from build123d import *

# Parameters (mm, degrees)
SKETCH1_W                               = 200
SKETCH1_H                               = 200
BOSS_EXTRUDE1_DEPTH                     = 8
CBORE_FOR_M2_PAN_HEAD_SCREW1_AT_2_COUNT = 2
CBORE_FOR_M2_PAN_HEAD_SCREW1_AT_2_PITCH = 89.990465529
CBORE_FOR_M2_PAN_HEAD_SCREW1_AT_3_COUNT = 2
CBORE_FOR_M2_PAN_HEAD_SCREW1_AT_3_PITCH = 89.990465529
CBORE_FOR_M2_PAN_HEAD_SCREW1_AT_4_COUNT = 2
CBORE_FOR_M2_PAN_HEAD_SCREW1_AT_4_PITCH = 66.987356945
CBORE_FOR_M2_PAN_HEAD_SCREW1_AT_5_COUNT = 2
CBORE_FOR_M2_PAN_HEAD_SCREW1_AT_5_PITCH = 23.002979742
SKETCH7_R                               = 2.5
CUT_EXTRUDE1_DEPTH                      = 4
SKETCH9_R                               = 1.5
CUT_EXTRUDE2_DEPTH                      = 10
LPATTERN1_COUNT                         = 2
LPATTERN1_PITCH                         = 100.5


with BuildPart() as part:
    # Sketch1 → Boss-Extrude1 (new body)
    with BuildSketch(Plane.XY):
        with Locations((100, 100)):
            Rectangle(SKETCH1_W, SKETCH1_H)
    extrude(amount=BOSS_EXTRUDE1_DEPTH)

    # Sketch6 → CBORE for M2 Pan Head Screw1 (revolve, cut)
    with BuildSketch(Plane(origin=(49.75, 55.009534471, 0), x_dir=(0, 1, 0), z_dir=(1, 0, 0))):
        Polygon((0, 0), (0, 8.901290929), (1.5, 8), (1.5, 4), (2.5, 4), (2.5, 0), align=None)
    cbore_for_m2_pan_head_screw1 = revolve(axis=Axis((49.75, 55.009534471, -6.35), (0, 0, 1)), mode=Mode.SUBTRACT)

    # CBORE for M2 Pan Head Screw1 at 2: CBORE for M2 Pan Head Screw1 ×2
    with Locations(*[(0, i * CBORE_FOR_M2_PAN_HEAD_SCREW1_AT_2_PITCH, 0) for i in range(1, CBORE_FOR_M2_PAN_HEAD_SCREW1_AT_2_COUNT)]):
        add(cbore_for_m2_pan_head_screw1, mode=Mode.SUBTRACT)

    # CBORE for M2 Pan Head Screw1 at 3: CBORE for M2 Pan Head Screw1 ×2
    with Locations(*[(0, i * CBORE_FOR_M2_PAN_HEAD_SCREW1_AT_3_PITCH, 0) for i in range(1, CBORE_FOR_M2_PAN_HEAD_SCREW1_AT_3_COUNT)]):
        add(cbore_for_m2_pan_head_screw1, mode=Mode.SUBTRACT)

    # CBORE for M2 Pan Head Screw1 at 4: CBORE for M2 Pan Head Screw1 ×2
    with Locations(*[(0, i * CBORE_FOR_M2_PAN_HEAD_SCREW1_AT_4_PITCH, 0) for i in range(1, CBORE_FOR_M2_PAN_HEAD_SCREW1_AT_4_COUNT)]):
        add(cbore_for_m2_pan_head_screw1, mode=Mode.SUBTRACT)

    # CBORE for M2 Pan Head Screw1 at 5: CBORE for M2 Pan Head Screw1 ×2
    with Locations(*[(0, i * CBORE_FOR_M2_PAN_HEAD_SCREW1_AT_5_PITCH, 0) for i in range(1, CBORE_FOR_M2_PAN_HEAD_SCREW1_AT_5_COUNT)]):
        add(cbore_for_m2_pan_head_screw1, mode=Mode.SUBTRACT)

    # Sketch7 → Cut-Extrude1 (cut)
    with BuildSketch(Plane(origin=(0, 0, 0), x_dir=(-1, 0, 0), z_dir=(0, 0, -1))):
        with Locations((-50, 100)):
            Circle(SKETCH7_R)
    cut_extrude1 = extrude(amount=-CUT_EXTRUDE1_DEPTH, mode=Mode.SUBTRACT)

    # Sketch9 → Cut-Extrude2 (cut)
    with BuildSketch(Plane(origin=(0, 0, 4), x_dir=(-1, 0, 0), z_dir=(0, 0, -1))):
        with Locations((-50, 100)):
            Circle(SKETCH9_R)
    cut_extrude2 = extrude(amount=-CUT_EXTRUDE2_DEPTH, mode=Mode.SUBTRACT)

    # LPattern1: CBORE for M2 Pan Head Screw1, Cut-Extrude1, Cut-Extrude2 ×2
    with Locations(*[(i * LPATTERN1_PITCH, 0, 0) for i in range(1, LPATTERN1_COUNT)]):
        add(cbore_for_m2_pan_head_screw1, mode=Mode.SUBTRACT)
        add(cut_extrude1, mode=Mode.SUBTRACT)
        add(cut_extrude2, mode=Mode.SUBTRACT)

    # LPattern1 copy 1 sketch → LPattern1 copy 1 (revolve, cut)
    with BuildSketch(Plane(origin=(150.25, 145, 0), x_dir=(0, 1, 0), z_dir=(1, 0, 0))):
        Polygon((0, 0), (0, 8.901290929), (1.5, 8), (1.5, 4), (2.5, 4), (2.5, 0), align=None)
    revolve(axis=Axis((150.25, 145, -6.35), (0, 0, 1)), mode=Mode.SUBTRACT)

    # LPattern1 copy 2 sketch → LPattern1 copy 2 (revolve, cut)
    with BuildSketch(Plane(origin=(150.25, 145, 0), x_dir=(0, 1, 0), z_dir=(1, 0, 0))):
        Polygon((0, 0), (0, 8.901290929), (1.5, 8), (1.5, 4), (2.5, 4), (2.5, 0), align=None)
    revolve(axis=Axis((150.25, 145, -6.35), (0, 0, 1)), mode=Mode.SUBTRACT)

    # LPattern1 copy 3 sketch → LPattern1 copy 3 (revolve, cut)
    with BuildSketch(Plane(origin=(150.25, 121.996891416, 0), x_dir=(0, 1, 0), z_dir=(1, 0, 0))):
        Polygon((0, 0), (0, 8.901290929), (1.5, 8), (1.5, 4), (2.5, 4), (2.5, 0), align=None)
    revolve(axis=Axis((150.25, 121.996891416, -6.35), (0, 0, 1)), mode=Mode.SUBTRACT)

    # LPattern1 copy 4 sketch → LPattern1 copy 4 (revolve, cut)
    with BuildSketch(Plane(origin=(150.25, 78.012514213, 0), x_dir=(0, 1, 0), z_dir=(1, 0, 0))):
        Polygon((0, 0), (0, 8.901290929), (1.5, 8), (1.5, 4), (2.5, 4), (2.5, 0), align=None)
    revolve(axis=Axis((150.25, 78.012514213, -6.35), (0, 0, 1)), mode=Mode.SUBTRACT)


solid = part.part
Can you work these out from the model? Positions are in its coordinate system, mm. A direction names the side the tool comes from. Give positions to 0.01 mm unless a question says otherwise; leave off trailing zeros. Write each question's results on one line, items separated by ' | '.
1) Please list where these lines run through material, in increasing order: line 1 along Y through (x, z) = (49.75, 0.9); line 2 along X through (y, z) = (145, 0.9); line 3 along X through (y, z) = (100, 7.25). Write a range as [from, to].
Final values:
line 1: y = [0, 52.51], [57.51, 75.51], [80.51, 97.51], [102.49, 119.5], [124.5, 142.5], [147.5, 200] | line 2: x = [0, 47.25], [52.25, 147.75], [152.75, 200] | line 3: x = [0, 48.5], [51.5, 149], [152, 200]
2) If we mould it in two halves opening along Y, with no side actions, what happens to faces 1 (the face through (99, 101, 0)), 2 (the face through (99, 200, 4)), 3 (the face through (49.64, 75.515, 1.972))? For each: pulls with the +Y half, pulls with the -Y half, needs draft (parallel to the pull), parting line crosses it, or undercut.
Final values:
face 1: needs draft | face 2: pulls with the +Y half | face 3: undercut
3) I'm going to push flat-ended pins straight in: pin 1 Ø1.8 at (x, y) = (150.25, 122) entering from +Z; pin 2 Ø4 at (x, y) = (149.5, 79) entering from -Z; pin 3 Ø4.5 at (x, y) = (49.75, 122) entering from -Z. Where does each tip first touch, or does it pass through?
Final values:
pin 1: passes through | pin 2: stops at z = 0 | pin 3: stops at z = 4
4) On a 3-axis mill with a long thin cutter (end or side, diameter ignored), from which of +Z, -Z, +X, -X, +Y, -Y can I reach the whole of each face in a straight line? I mean faces 4 (the face through (99, 101, 8)), 5 (the face through (147.77, 54.68, 1.97)). Say none if no direction works.
Final values:
face 4: +Z, +X, -X, +Y, -Y | face 5: -Z
